from build123d import *

# Parameters (mm, degrees)
BOSS_EXTRUDE1_DEPTH      = 75
BOSS_EXTRUDE1_DEPTH_BACK = 75
BOSS_EXTRUDE2_START      = -10
SKETCH2_R                = 6.3
BOSS_EXTRUDE2_DEPTH      = 10
SKETCH3_R                = 6.3
BOSS_EXTRUDE3_DEPTH      = 10
SKETCH4_R                = 1.1
CUT_EXTRUDE1_DEPTH       = 84.216584885
SKETCH5_R                = 2.1
CUT_EXTRUDE2_DEPTH       = 87.168439698
CUT_EXTRUDE3_DEPTH       = 6
FILLET1_R                = 4
FILLET2_R                = 4
FILLET3_R                = 32
BOSS_EXTRUDE4_DEPTH      = 12
BOSS_EXTRUDE5_START      = -43.5
BOSS_EXTRUDE5_DEPTH      = 12
BOSS_EXTRUDE7_START      = 44
BOSS_EXTRUDE7_DEPTH      = 12
SKETCH16_R               = 13
CUT_EXTRUDE8_DEPTH       = 99.5


with BuildPart() as part:
    # Sketch1 → Boss-Extrude1 (new, two sides: drawn at the far end of the back side and taken through both)
    with BuildSketch(Plane(origin=(0, 0, 0), x_dir=(0, 0, -1), z_dir=(1, 0, 0)).offset(-BOSS_EXTRUDE1_DEPTH_BACK)):
        with BuildLine():
            Line((-12.649110641, -6), (-30, -6))
            Line((-30, -6), (-30, -16))
            Line((-30, -16), (30, -16))
            Line((30, -16), (30, -6))
            Line((30, -6), (12.649110641, -6))
            ThreePointArc((12.649110641, -6), (0, -14), (-12.649110641, -6))
        make_face()
    extrude(amount=BOSS_EXTRUDE1_DEPTH + BOSS_EXTRUDE1_DEPTH_BACK)

    # Sketch2 → Boss-Extrude2 (add)
    with BuildSketch(Plane(origin=(75, 0, 0), x_dir=(0, 0, -1), z_dir=(1, 0, 0)).offset(BOSS_EXTRUDE2_START)):
        with BuildLine():
            Line((-14, 0), (-14, -16))
            Line((-14, -16), (14, -16))
            Line((14, -16), (14, 0))
            ThreePointArc((14, 0), (0, 14), (-14, 0))
        make_face()
        Circle(SKETCH2_R, mode=Mode.SUBTRACT)
    extrude(amount=BOSS_EXTRUDE2_DEPTH)

    # Sketch3 → Boss-Extrude3 (add)
    with BuildSketch(Plane.ZY.offset(75)):
        with BuildLine():
            Line((-14, 0), (-14, -16))
            Line((-14, -16), (14, -16))
            Line((14, -16), (14, 0))
            ThreePointArc((14, 0), (0, 14), (-14, 0))
        make_face()
        with Locations(Location((0, 0, 0), (0, 0, 180))):
            Circle(SKETCH3_R, mode=Mode.SUBTRACT)
    extrude(amount=-BOSS_EXTRUDE3_DEPTH)

    # Sketch4 → Cut-Extrude1 (cut, through all)
    with BuildSketch(Plane(origin=(0, -6, 0), x_dir=(1, 0, 0), z_dir=(0, 1, 0))):
        with Locations(Location((-15.4853, -16, 0), (0, 0, 270))):
            Circle(SKETCH4_R)
        with Locations(Location((-59.1364, 16, 0), (0, 0, 270))):
            Circle(SKETCH4_R)
        with Locations(Location((28.1658, 16, 0), (0, 0, 270))):
            Circle(SKETCH4_R)
    extrude(amount=-CUT_EXTRUDE1_DEPTH, mode=Mode.SUBTRACT)

    # Sketch5 → Cut-Extrude2 (cut, through all)
    with BuildSketch(Plane.XZ.offset(16)):
        with Locations(Location((-35, 25, 0), (0, 0, 270))):
            Circle(SKETCH5_R)
        with Locations(Location((35, 25, 0), (0, 0, 270))):
            Circle(SKETCH5_R)
        with Locations(Location((-20, -25, 0), (0, 0, 270))):
            Circle(SKETCH5_R)
        with Locations(Location((20, -25, 0), (0, 0, 270))):
            Circle(SKETCH5_R)
    extrude(amount=-CUT_EXTRUDE2_DEPTH, mode=Mode.SUBTRACT)

    # Sketch7 → Cut-Extrude3 (cut)
    with BuildSketch(Plane.XZ.offset(16)):
        Polygon((-37.078460969, 28.6), (-39.156921938, 25), (-37.078460969, 21.4), (-32.921539031, 21.4), (-30.843078062, 25), (-32.921539031, 28.6), align=None)
        Polygon((32.921539031, 28.6), (30.843078062, 25), (32.921539031, 21.4), (37.078460969, 21.4), (39.156921938, 25), (37.078460969, 28.6), align=None)
        Polygon((-22.078460969, -21.4), (-24.156921938, -25), (-22.078460969, -28.6), (-17.921539031, -28.6), (-15.843078062, -25), (-17.921539031, -21.4), align=None)
        Polygon((17.921539031, -21.4), (15.843078062, -25), (17.921539031, -28.6), (22.078460969, -28.6), (24.156921938, -25), (22.078460969, -21.4), align=None)
    extrude(amount=-CUT_EXTRUDE3_DEPTH, mode=Mode.SUBTRACT)

    # Fillet1
    fillet1_edges = [part.edges().sort_by_distance(p)[0] for p in [
        (70, -6, -14),
        (70, -6, 14),
        (-70, -6, 14),
        (-70, -6, -14),
    ]]
    fillet(fillet1_edges, radius=FILLET1_R)

    # Fillet2
    fillet2_edges = [part.edges().sort_by_distance(p)[0] for p in [
        (-75, -11, -30),
        (75, -11, -30),
    ]]
    fillet(fillet2_edges, radius=FILLET2_R)

    # Fillet3
    # the kernel refuses this fillet: 32 mm, written as the material it takes off along each edge
    with BuildSketch(Plane(origin=(75, 74, 30), x_dir=(0, 0, -1), z_dir=(0, -1, 0)), Plane(origin=(-75, 74, 30), x_dir=(1, 0, 0), z_dir=(0, -1, 0))) as fillet3_piece_1:
        with BuildLine():
            CenterArc((FILLET3_R, -FILLET3_R), FILLET3_R, 90, 90)
            Line((0, -FILLET3_R), (0, 0))
            Line((0, 0), (FILLET3_R, 0))
        make_face()
    extrude(amount=170, mode=Mode.SUBTRACT)

    # Sketch8 → Boss-Extrude4 (add)
    with BuildSketch(Plane.ZY.offset(21)):
        with BuildLine():
            Line((-10.9658561, -6), (-13.747727085, -6))
            ThreePointArc((-13.747727085, -6), (0, -15), (13.747727085, -6))
            Line((13.747727085, -6), (10.9658561, -6))
            ThreePointArc((10.9658561, -6), (0, -12.5), (-10.9658561, -6))
        make_face()
    extrude(amount=-BOSS_EXTRUDE4_DEPTH)

    # Sketch8<2> → Boss-Extrude5 (add)
    with BuildSketch(Plane.ZY.offset(21).offset(BOSS_EXTRUDE5_START)):
        with BuildLine():
            Line((-10.9658561, -6), (-13.747727085, -6))
            ThreePointArc((-13.747727085, -6), (0, -15), (13.747727085, -6))
            Line((13.747727085, -6), (10.9658561, -6))
            ThreePointArc((10.9658561, -6), (0, -12.5), (-10.9658561, -6))
        make_face()
    extrude(amount=-BOSS_EXTRUDE5_DEPTH)

    # Sketch8<4> → Boss-Extrude7 (add)
    with BuildSketch(Plane.ZY.offset(21).offset(BOSS_EXTRUDE7_START)):
        with BuildLine():
            Line((-10.9658561, -6), (-13.747727085, -6))
            ThreePointArc((-13.747727085, -6), (0, -15), (13.747727085, -6))
            Line((13.747727085, -6), (10.9658561, -6))
            ThreePointArc((10.9658561, -6), (0, -12.5), (-10.9658561, -6))
        make_face()
    extrude(amount=-BOSS_EXTRUDE7_DEPTH)

    # Sketch16 → Cut-Extrude8 (cut)
    with BuildSketch(Plane(origin=(-65, 0, 0), x_dir=(0, 0, -1), z_dir=(1, 0, 0))):
        Circle(SKETCH16_R)
    extrude(amount=CUT_EXTRUDE8_DEPTH, mode=Mode.SUBTRACT)


solid = part.part
Input: part model. Units: mm. Frame: model coordinates. A direction names the side the tool comes from. Coordinates: 2 decimals unless noted, no trailing zeros. Loops run counter-clockwise (first coordinate to the right, second up) from the corner with the lowest first, then second, coordinate; pieces in that order, holes last.
(1) Section A-A on x = 20. Return the cut outline in (y, z), then the cut area to 3 significant figures.
(2) Section B-B on z = 3. Return the cut outline in (x, y), then the cut area to 3 significant figures.
(3) Section D-D on x = 0.5. Return the cut outline in (y, z), then the cut area to 3 significant figures.
(4) Section C-C on z = -9. Return the cut outline in (x, y), then the cut area to 3 significant figures.
(5) Set-up query: faces 4 (the face through (-18.23, -8.03, -26.13)), 5 (the face through (34.5, -13.2, -0.1)), 6 (the face through (23, -13, -27)). Return all of +Z, -Z, +X, -X, +Y, -Y with unobstructed straight access to the full face (end or side cutting, diameter ignored); none if empty.
(6) Pull-direction query (Z, two-part tool) for faces 1 (the face through (-73.797, -10.93, -28.859)), 2 (the face through (20.631, -8.028, -27.003)), 3 (the face through (-1, -16, 0)); classes: released by +Z, released by -Z, zero draft, split by the parting line, or undercut.
(7) Material intervals for probe 1 along X at (y, z) = (-8.35, -25); probe 2 along X at (y, z) = (-13.5, -16); probe 3 along Y at (x, z) = (-70, 0), sorted ascending.
(8) First-contact query: pin 1 Ø2 at (x, z) = (37, 23.5) entering from -Y; pin 2 Ø3.5 at (x, z) = (35, 25) entering from -Y; pin 3 Ø2 at (x, y) = (-68.5, -1) entering from +Z; pin 4 Ø14.5 at (y, z) = (0, 0) entering from -X. Flat tips, straight axial feed; report the tip coordinate or a pass-through.
Data:
1. outline: (-16, -30) - (-6, -30) - (-6, -27.1) - (-10, -27.1) - (-10, -28.6) - (-16, -28.6) - close; (-16, -21.4) - (-10, -21.4) - (-10, -22.9) - (-6, -22.9) - (-6, -12.65) arc R14 cw to (-6, 12.65) - (-6, 30) - (-16, 30) - close
1. area: 395 mm2
2. outline: (-74.61, -16) - (74.61, -16) - (74.61, -5.54) - (65, -5.54) - (65, -13.67) - (34.5, -13.67) - (34.5, -12.65) - (22.5, -12.65) - (22.5, -13.67) - (-9, -13.67) - (-9, -12.65) - (-21, -12.65) - (-21, -13.67) - (-53, -13.67) - (-53, -12.65) - (-65, -12.65) - (-65, -5.54) - (-74.61, -5.54) - close; (-74.61, 5.54) - (-65, 5.54) - (-65, 13.67) - (-74.61, 13.67) - close; (65, 5.54) - (74.61, 5.54) - (74.61, 13.67) - (65, 13.67) - close
2. area: 696 mm2
3. outline: (-16, -30) - (-6, -30) - (-6, -12.65) arc R14 cw to (-6, 12.65) - (-6, 30) - (-16, 30) - close
3. area: 455 mm2
4. outline: (-75, -16) - (75, -16) - (75, 10.72) - (65, 10.72) - (65, -10.72) - (34.5, -10.72) - (34.5, -9.38) - (22.5, -9.38) - (22.5, -10.72) - (-9, -10.72) - (-9, -9.38) - (-21, -9.38) - (-21, -10.72) - (-53, -10.72) - (-53, -9.38) - (-65, -9.38) - (-65, 10.72) - (-75, 10.72) - close
4. area: 1,270 mm2
5. face 4: +Y, -Y
5. face 5: +Y
5. face 6: -Y
6. face 1: released by -Z
6. face 2: undercut
6. face 3: zero draft
7. probe 1: x = -75 to -22.1, -17.9 to 17.9, 22.1 to 75
7. probe 2: x = -75 to -60.24, -58.04 to 27.07, 29.27 to 75
7. probe 3: y = -16 to -6.3, 6.3 to 14
8. pin 1: stops at y = -10
8. pin 2: passes through
8. pin 3: stops at z = 14
8. pin 4: stops at x = -75
